```python
from build123d import *

# Parameters (mm, degrees)
BOX_W          = 3.2
BOX_H          = 10
BOX_DEPTH      = 4
ARRAY_COUNT    = 4
CYLINDER_R     = 17
CYLINDER_DEPTH = 2


with BuildPart() as array:
    # Box → Box (new body)
    with BuildSketch(Plane(origin=(-1.6, 9, -1), x_dir=(1, 0, 0), z_dir=(0, 0, 1))):
        with Locations((1.6, 5)):
            Rectangle(BOX_W, BOX_H)
    extrude(amount=BOX_DEPTH)

    # Array: Array ×4 about axis
    array_axis = Axis((0, 0, 0), (0, 0, 1))


with BuildPart() as array_1:
    add(array.part)
    for i in range(1, ARRAY_COUNT):
        add(array.part.rotate(array_axis, i * 360 / ARRAY_COUNT))


with BuildPart() as cut:
    # Cylinder → Cylinder (new body)
    with BuildSketch(Plane.XY):
        Circle(CYLINDER_R)
    extrude(amount=CYLINDER_DEPTH)

    # Cut: cut Array
    add(array_1.part, mode=Mode.SUBTRACT)


solid = cut.part
```
Can you work these out from the model? Positions are in its coordinate system, mm. A direction names the side the tool comes from. Coordinates: 2 decimals unless noted, no trailing zeros. Loops run counter-clockwise (first coordinate to the right, second up) from the corner with the lowest first, then second, coordinate; pieces in that order, holes last.
1) Imagine slicing it at D-D on y = -0.5. List the corners of the cut face in (x, z) for me, plus the area to 3 significant figures.
2) Thinking about a two-plate mould opening in X: for faces 1 (the flat face through (13, -1.6, 1)), 2 (the cylindrical face through (12.14, 11.9, 0.99)), 3 (the flat face through (-1.6, -13, 1)), which applies, pulls with the +X half, pulls with the -X half, needs draft (parallel to the pull), parting line crosses it, or undercut?
3) Imagine slicing it at C-C on y = 13. List the corners of the cut face in (x, z) for me.
4) Which directions (+Z, -Z, +X, -X, +Y, -Y) give clear straight access to the entire face, cutting with the end or side of a thin tool? Please do faces 4 (the flat face through (0, 9, 1)), 5 (the flat face through (-9, 0, 1)), 6 (the flat face through (1.6, -13, 1)), 7 (the flat face through (13, 1.6, 1)).
5) I need wall thicknesses on probe 1 along X at (y, z) = (15, 1.65); probe 2 along X at (y, z) = (13, 1.6); probe 3 along Y at (x, z) = (0, 0.25). Which ranges of each line are inside material? Lowest first, please.
6) For pin 1 (1 mm diameter, centred on x = -13, z = 1, fed in from +Y); pin 2 (1 mm diameter, centred on x = -0.5, z = 1, fed in from +Y); pin 3 (0.6 mm diameter, centred on y = 14, z = 1, fed in from +X), each with a flat end and sliding along its axis, tell me the tip position at first contact or that it passes through.
7) Imagine slicing it at B-B on z = 0.5. List the corners of the cut face in (x, y) for me, plus the area to 3 significant figures.
8) Imagine slicing it at A-A on x = 15. List the corners of the cut face in (y, z) for me, plus the area to 3 significant figures.
Completed:
1. outline: (-9, 0) - (9, 0) - (9, 2) - (-9, 2) - close
1. area: 36.0 mm2
2. face 1: needs draft
2. face 2: pulls with the +X half
2. face 3: undercut
3. outline: (-10.95, 0) - (-1.6, 0) - (-1.6, 2) - (-10.95, 2) - close; (1.6, 0) - (10.95, 0) - (10.95, 2) - (1.6, 2) - close
4. face 4: +Z, -Z, +Y
4. face 5: +Z, -Z, -X
4. face 6: +Z, -Z, -Y
4. face 7: +Z, -Z, +X
5. probe 1: x = -8 to -1.6, 1.6 to 8
5. probe 2: x = -10.95 to -1.6, 1.6 to 10.95
5. probe 3: y = -9 to 9
6. pin 1: stops at y = 11.52
6. pin 2: stops at y = 9
6. pin 3: stops at x = 10.07
7. outline: (-16.92, -1.6) arc R17 ccw to (-1.6, -16.92) - (-1.6, -9) - (1.6, -9) - (1.6, -16.92) arc R17 ccw to (16.92, -1.6) - (9, -1.6) - (9, 1.6) - (16.92, 1.6) arc R17 ccw to (1.6, 16.92) - (1.6, 9) - (-1.6, 9) - (-1.6, 16.92) arc R17 ccw to (-16.92, 1.6) - (-9, 1.6) - (-9, -1.6) - close
7. area: 806 mm2
8. outline: (-8, 0) - (-1.6, 0) - (-1.6, 2) - (-8, 2) - close; (1.6, 0) - (8, 0) - (8, 2) - (1.6, 2) - close
8. area: 25.6 mm2
